The figure shows three views and two pictorial views of one solid part (mm, origin at its lowest corner). Answer the questions. Round coordinates to 2 decimals unless told otherwise and drop trailing zeros. Order: outer loops, then holes, each group sorted by start corner. A loop starts at its lowest first (then second) coordinate and runs counter-clockwise, first axis right, second up. Notation, with made-up numbers: (-8, 56) - (-4, 56) arc R7 ccw to (-4, 60) - close; hole circle Ø11 at (-18.75, 89.25). An arc over 180 degrees is marked (long way). Answer in a Markdown table with one row per item.
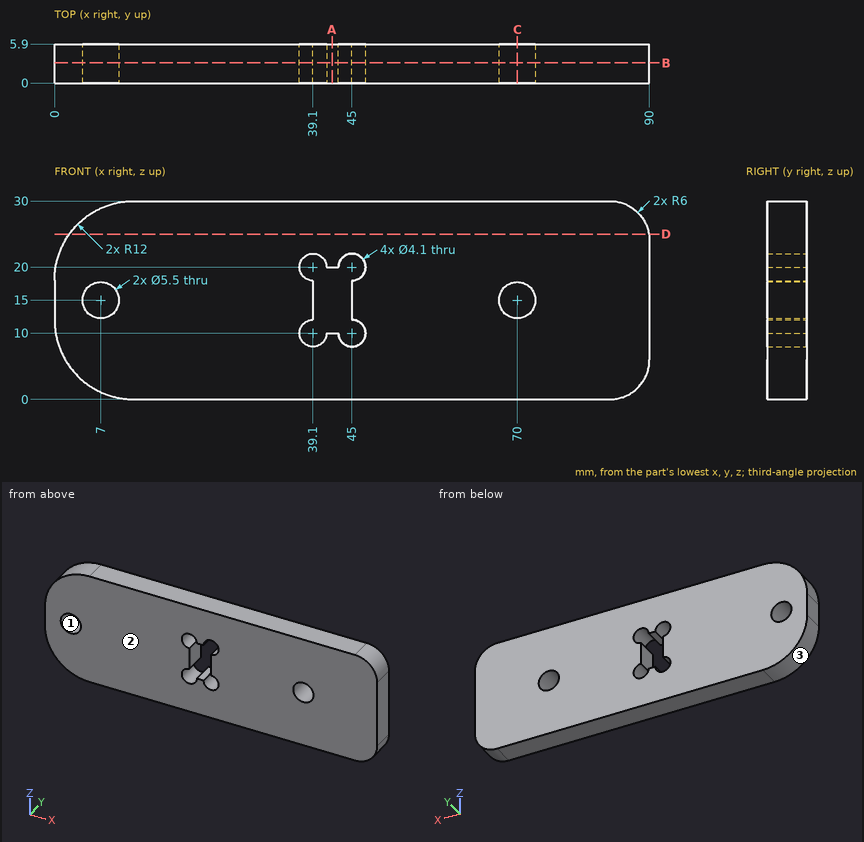
1) Find section C-C, the plane x = 70. Give the vertices of the cut face in (y, z), then the cut area to 3 significant figures.
Filled in:
| item | result |
|---|---|
| outline | (0, 0) - (5.9, 0) - (5.9, 12.25) - (0, 12.25) - close; (0, 17.75) - (5.9, 17.75) - (5.9, 30) - (0, 30) - close |
| area | 145 mm^2 |
2) Find section B-B, the plane y = 3.05. Give the vertices of the cut face in (x, z).
Filled in:
| item | result |
|---|---|
| outline | (0, 12) arc R12 ccw to (12, 0) - (84, 0) arc R6 ccw to (90, 6) - (90, 24) arc R6 ccw to (84, 30) - (12, 30) arc R12 ccw to (0, 18) - close; hole circle Ø5.5 at (7, 15); hole (39.1, 12.05) arc R2.05 ccw (long way) to (41.15, 10) - (42.95, 10) arc R2.05 ccw (long way) to (45, 12.05) - (45, 17.95) arc R2.05 ccw (long way) to (42.95, 20) - (41.15, 20) arc R2.05 ccw (long way) to (39.1, 17.95) - close; hole circle Ø5.5 at (70, 15) |
3) Find the intervals of material crossed by probe 1 along X at (y, z) = (2.95, 13.5); probe 2 along Z at (x, y) = (7, 4); probe 3 along X at (y, z) = (3.5, 11), in increasing order. Write a range as from..to.
Filled in:
| item | result |
|---|---|
| probe 1 | x = 0..4.7, 9.3..39.1, 45..67.7, 72.3..90 |
| probe 2 | z = 1.09..12.25, 17.75..28.91 |
| probe 3 | x = 0.04..37.31, 46.79..90 |
4) The mould has two halves that part along X. Classify the marked faces 1, 2 and 3: released by +X, released by -X, zero draft, split by the parting line, or undercut.
Filled in:
| item | result |
|---|---|
| face 1 | undercut |
| face 2 | zero draft |
| face 3 | released by -X |
5) This flat-tipped pin is pushed along its axis until it touches: pin 1 (10 mm diameter, centred on x = 63.5, z = 10.5, fed in from -Y). Where does it stop, or does it pass through?
Filled in:
| item | result |
|---|---|
| pin 1 | stops at y = 0 |
6) Find section A-A, the plane x = 42. Give the vertices of the cut face in (y, z).
Filled in:
| item | result |
|---|---|
| outline | (0, 0) - (5.9, 0) - (5.9, 10) - (0, 10) - close; (0, 20) - (5.9, 20) - (5.9, 30) - (0, 30) - close |
7) Find section D-D, the plane z = 25. Give the vertices of the cut face in (x, y), then the cut area to 3 significant figures.
Filled in:
| item | result |
|---|---|
| outline | (2.25, 0) - (89.92, 0) - (89.92, 5.9) - (2.25, 5.9) - close |
| area | 517 mm^2 |
